```python
from build123d import *

# Parameters (mm, degrees)
F0_W      = 304.8
F0_H      = 152.4
F1_DEPTH  = 50.8
F2_W      = 152.4
F2_H      = 19.05
F4_W      = 12.7
F4_H      = 5.08
F5_DEPTH  = 25.4
F6_W      = 76.2
F6_H      = 7.62
F9_W      = 228.6
F9_H      = 63.5
F9_W_2    = 14.362933135
F10_DEPTH = 6.35
F8_W      = 6.35
F8_H      = 152.4
F8_W_2    = 44.45
F11_DEPTH = 76.2
F12_W     = 71.5284022924
F12_H     = 63.5
F13_DEPTH = 6.35
F14_R     = 3.175
F15_DEPTH = 12.7
F16_W     = 381
F16_H     = 50.8
F17_DEPTH = 50.8
F18_W     = 304.8
F18_H     = 44.45
F19_DEPTH = 6.35
F20_R     = 3.175
F21_DEPTH = 19.05
F22_W     = 71.1707984924
F22_H     = 12.7
F24_DEPTH = 6.35


with BuildPart() as f1:
    # F0 (on Front) → F1 (new body)
    with BuildSketch(Plane.XZ):
        with Locations((-5.0292015076, 4.4291064884)):
            Rectangle(F0_W, F0_H)
    extrude(amount=F1_DEPTH)

    # F2 (on face) → F3 (revolve, cut)
    with BuildSketch(Plane.XZ.offset(50.8)):
        with Locations((-76.2, -9.525)):
            Rectangle(F2_W, F2_H)
    revolve(axis=Axis((-76.2, -50.8, 0), (-1, 0, 0)), mode=Mode.SUBTRACT)

    # F4 (on face) → F5 (cut)
    with BuildSketch(Plane.XZ.offset(50.8)):
        with Locations((-38.1, 2.54)):
            Rectangle(F4_W, F4_H)
        with Locations((-38.1, -2.54)):
            Rectangle(F4_W, F4_H)
    extrude(amount=-F5_DEPTH, mode=Mode.SUBTRACT)

    # F6 (on face) → F7 (revolve, cut)
    with BuildSketch(Plane.XZ.offset(50.8)):
        with Locations((38.1, -3.81)):
            Rectangle(F6_W, F6_H)
    revolve(axis=Axis((38.1, -50.8, 0), (1, 0, 0)), mode=Mode.SUBTRACT)

    # F9 (on face) → F10 (cut)
    with BuildSketch(Plane.XZ.offset(50.8)):
        with Locations((-38.1, -34.6967290044)):
            Rectangle(F9_W, F9_H)
        with Locations((-159.5814665675, -34.6967290044)):
            Rectangle(F9_W_2, F9_H)
    extrude(amount=-F10_DEPTH, mode=Mode.SUBTRACT)

    # F8 (on face) → F11 (join)
    with BuildSketch(Plane(origin=(-157.4292015076, 0, 0), x_dir=(0, -1, 0), z_dir=(-1, 0, 0))):
        with Locations((47.625, 4.4291064884)):
            Rectangle(F8_W, F8_H)
        with Locations((22.225, 4.4291064884)):
            Rectangle(F8_W_2, F8_H)
    extrude(amount=F11_DEPTH)

    # F12 (on face) → F13 (cut)
    with BuildSketch(Plane.XZ.offset(50.8)):
        with Locations((-193.1934026538, -34.6967290044)):
            Rectangle(F12_W, F12_H)
    extrude(amount=-F13_DEPTH, mode=Mode.SUBTRACT)

    # F14 (on face) → F15 (join)
    with BuildSketch(Plane.XZ.offset(44.45)):
        with Locations((-152.4, -60.3105122421)):
            Circle(F14_R)
    extrude(amount=F15_DEPTH)

    # F16 (on face) → F17 (join)
    with BuildSketch(Plane(origin=(0, 0, -71.7708935116), x_dir=(1, 0, 0), z_dir=(0, 0, -1))):
        with Locations((-43.1292015076, 25.4)):
            Rectangle(F16_W, F16_H)
    extrude(amount=F17_DEPTH)

    # F18 (on face) → F19 (cut)
    with BuildSketch(Plane.XZ.offset(50.8)):
        with Locations((-76.5576038, -88.6717290044)):
            Rectangle(F18_W, F18_H)
    extrude(amount=-F19_DEPTH, mode=Mode.SUBTRACT)

    # F20 (on face) → F21 (join)
    with BuildSketch(Plane.XZ.offset(44.45)):
        with Locations((-106.7121654678, -85.4967290044)):
            Circle(F20_R)
    extrude(amount=F21_DEPTH)

    # F22 (on face) → F23 (revolve, cut)
    with BuildSketch(Plane.XZ.offset(50.8)):
        with Locations((111.7853992462, -6.35)):
            Rectangle(F22_W, F22_H)
    revolve(axis=Axis((111.7853992462, -50.8, 0), (1, 0, 0)), mode=Mode.SUBTRACT)

    # F14 (on face) → F24 (join)
    with BuildSketch(Plane.XZ.offset(44.45)):
        with Locations((-152.4, -60.3105122421)):
            Circle(F14_R)
    extrude(amount=F24_DEPTH)


solid = f1.part
```
CAD build for the part. Positions are in the model's coordinates, mm. A direction names the side the tool comes from. Give positions to 0.01 mm unless a question says otherwise; leave off trailing zeros. Order: outer loops, then holes, each group sorted by start corner. A loop starts at its lowest first (then second) coordinate and runs counter-clockwise, first axis right, second up.
(1) Flat gauge pins, fed straight in: pin 1 (4 mm diameter, centred on x = -165, z = 58, fed in from +Y); pin 2 (8 mm diameter, centred on x = -37.5, z = 1.5, fed in from -Y); pin 3 (10 mm diameter, centred on y = -44.5, z = -0.5, fed in from +X); pin 4 (1.9 mm diameter, centred on x = -151.5, z = -60.5, fed in from -Y). Where does each tip first touch, or does it go through?
(2) Mould opens along Z. For faces 1 (the flat face through (-40, -26, 80.629)), 2 (the flat face through (-44.45, -29, 0)), 3 (the cylindrical face through (38.63, -44.03, 3.5)), 4 (the flat face through (-46, 0, -20)) say: released by +Z, released by -Z, zero draft, split by the parting line, or undercut.
(3) Drill centre lines: L1, parallel to Z at x = -11.5, y = -50.5; L2, parallel to Y at x = 93.5, z = -22; L3, parallel to Y at x = -18, z = -110. Where is each one in solid material? Low to high.
(4) Saw through at A-A, the plane x = 11.5. Give the cut face in (y, z), then the cut area to 3 significant figures.
(5) Tool access for faces 5 (the flat face through (76.2, -43, 1)), 6 (the flat face through (-233.629, -25, -20)), 7 (the flat face through (-31.75, -29, 0)): list every direction of +Z, -Z, +X, -X, +Y, -Y with a clear straight run to the whole face (end or side of a thin tool).
(6) Saw through at B-B, the plane x = -189. Give the cut face in (y, z), then the cut area to 3 significant figures.
Results found:
1. pin 1: stops at y = 0
1. pin 2: stops at y = -32.56
1. pin 3: stops at x = 76.2
1. pin 4: stops at y = -57.15
2. face 1: released by +Z
2. face 2: undercut
2. face 3: undercut
2. face 4: zero draft
3. L1: z = -122.57 to -110.9, 19.05 to 80.63
3. L2: y = -50.8 to 0
3. L3: y = -44.45 to 0
4. outline: (-50.8, -122.57) - (0, -122.57) - (0, 80.63) - (-50.8, 80.63) - (-50.8, 7.62) arc R7.62 cw to (-44.45, -4.21) - (-44.45, -110.9) - (-50.8, -110.9) - close
4. area: 9,570 mm2
5. face 5: +X, -Y
5. face 6: +Z, -Z, -X, +Y, -Y
5. face 7: -Y
6. outline: (-50.8, -122.57) - (0, -122.57) - (0, 80.63) - (-50.8, 80.63) - (-50.8, -2.95) - (-44.45, -2.95) - (-44.45, -110.9) - (-50.8, -110.9) - close
6. area: 9,640 mm2
